Verification items for the finished model (mm, model axes). Give positions to 0.01 mm unless a question says otherwise; leave off trailing zeros. Order: outer loops, then holes, each group sorted by start corner. A loop starts at its lowest first (then second) coordinate and runs counter-clockwise, first axis right, second up. Notation, with made-up numbers: M 10,86 L 38,86 A29 ccw 38,109 Z; hole C 59.25,43 d9. An arc over 180 degrees is marked long. Answer as a JSON object with one key per item and string values.
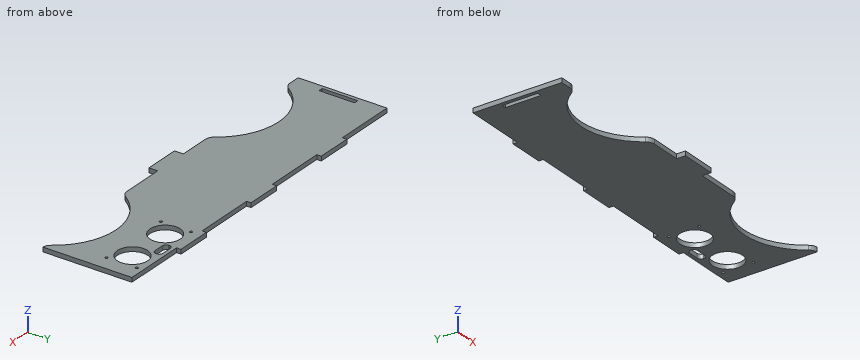
```python
from build123d import *

# Parameters (mm, degrees)
SKETCH1_R           = 8.5
SKETCH1_R_2         = 0.75
SKETCH1_W           = 2.5
SKETCH1_H           = 20
BOSS_EXTRUDE1_DEPTH = 1.25
FILLET2_R           = 5


with BuildPart() as part:
    # Sketch1 → Boss-Extrude1 (new, symmetric)
    with BuildSketch(Plane.XY):
        with BuildLine():
            Line((-100, -25), (-100, 25))
            Line((-100, 25), (-65, 25))
            Line((-65, 25), (-65, 27.5))
            Line((-65, 27.5), (-45, 27.5))
            Line((-45, 27.5), (-45, 25))
            Line((-45, 25), (-10, 25))
            Line((-10, 25), (-10, 27.5))
            Line((-10, 27.5), (10, 27.5))
            Line((10, 27.5), (10, 25))
            Line((10, 25), (45, 25))
            Line((45, 25), (45, 27.5))
            Line((45, 27.5), (65, 27.5))
            Line((65, 27.5), (65, 25))
            Line((65, 25), (100, 25))
            Line((100, 25), (100, -25))
            Line((100, -25), (97.62, -25))
            ThreePointArc((97.62, -25), (67.309110868, -7.5), (36.998221735, -25))
            Line((36.998221735, -25), (10, -25))
            Line((10, -25), (10, -30))
            Line((10, -30), (-10, -30))
            Line((-10, -30), (-10, -25))
            Line((-10, -25), (-30.118221735, -25))
            ThreePointArc((-30.118221735, -25), (-60.429110868, -7.5), (-90.74, -25))
            Line((-90.74, -25), (-100, -25))
        make_face()
        with Locations((57.2, 13)):
            Circle(SKETCH1_R, mode=Mode.SUBTRACT)
        with Locations((48.75, 4.5)):
            Circle(SKETCH1_R_2, mode=Mode.SUBTRACT)
        with Locations(Location((91.25, 4.5, 0), (0, 0, 180))):
            Circle(SKETCH1_R_2, mode=Mode.SUBTRACT)
        with Locations(Location((82.8, 13, 0), (0, 0, 180))):
            Circle(SKETCH1_R, mode=Mode.SUBTRACT)
        with Locations((91.25, 21.5)):
            Circle(SKETCH1_R_2, mode=Mode.SUBTRACT)
        with Locations(Location((48.75, 21.5, 0), (0, 0, 180))):
            Circle(SKETCH1_R_2, mode=Mode.SUBTRACT)
        with Locations((-96.75, 0)):
            Rectangle(SKETCH1_W, SKETCH1_H, mode=Mode.SUBTRACT)
        with BuildLine():
            Line((67, 18.6), (73, 18.6))
            ThreePointArc((73, 18.6), (74.414213562, 19.185786438), (75, 20.6))
            Line((75, 20.6), (75, 21))
            ThreePointArc((75, 21), (74.414213562, 22.414213562), (73, 23))
            Line((73, 23), (67, 23))
            ThreePointArc((67, 23), (65.585786438, 22.414213562), (65, 21))
            Line((65, 21), (65, 20.6))
            ThreePointArc((65, 20.6), (65.585786438, 19.185786438), (67, 18.6))
        make_face(mode=Mode.SUBTRACT)
    extrude(amount=BOSS_EXTRUDE1_DEPTH, both=True)

    # Fillet2
    # the kernel refuses this fillet: 5 mm, written as the material it takes off along each edge
    with BuildSketch(Plane(origin=(97.62, -25, 7.66613531), x_dir=(-0.5314154668172085, 0.8471113277648036, 0), z_dir=(0, 0, -1))) as fillet2_piece_1:
        with BuildLine():
            CenterArc((2.749772276, 4.996638315), FILLET2_R, 216.591278999, 51.307578807)
            Line((-1.264768811, 2.01612496), (-1.345059633, 1.956514693))
            ThreePointArc((-1.345059633, 1.956514693), (-0.717095538, 0.954920933), (-0.084711133, -0.053141547))
            Line((-0.084711133, -0.053141547), (0.003666363, -0.099932766))
            ThreePointArc((0.003666363, -0.099932766), (1.283227062, -0.076468208), (2.562787761, -0.099932766))
            Line((2.562787761, -0.099932766), (2.566454124, 0))
        make_face()
    extrude(amount=15.332270621, mode=Mode.SUBTRACT)
    with BuildSketch(Plane(origin=(36.998221735, -25, 8.15250564), x_dir=(-1, 0, 0), z_dir=(0, 0, -1)), Plane(origin=(-30.118221735, -25, -8.15250564), x_dir=(1, 0, 0), z_dir=(0, 0, 1))) as fillet2_piece_2:
        with BuildLine():
            CenterArc((2.761002256, 5), FILLET2_R, 214.228866328, 55.771133672)
            Line((-1.372984168, 2.1875), (-1.455663896, 2.13125))
            ThreePointArc((-1.455663896, 2.13125), (-0.751006819, 1.053257332), (-0.08660254, -0.05))
            Line((-0.08660254, -0.05), (0, -0.1))
            Line((0, -0.1), (2.761002256, -0.1))
            Line((2.761002256, -0.1), (2.761002256, 0))
        make_face()
    extrude(amount=16.305011279, mode=Mode.SUBTRACT)
    with BuildSketch(Plane(origin=(-90.74, -25, -8.15250564), x_dir=(-1, 0, 0), z_dir=(0, 0, 1))) as fillet2_piece_3:
        with BuildLine():
            CenterArc((2.761002256, -5), FILLET2_R, 90, 55.771133672)
            Line((-1.372984168, -2.1875), (-1.455663896, -2.13125))
            ThreePointArc((-1.455663896, -2.13125), (-0.751006819, -1.053257332), (-0.08660254, 0.05))
            Line((-0.08660254, 0.05), (0, 0.1))
            Line((0, 0.1), (2.761002256, 0.1))
            Line((2.761002256, 0.1), (2.761002256, 0))
        make_face()
    extrude(amount=16.305011279, mode=Mode.SUBTRACT)


solid = part.part
```
Q1. Material ranges on L1, parallel to X at y = -15, z = -0.7; L2, parallel to X at y = -22.5, z = -0.4; L3, parallel to Y at x = 13, z = -0.1, recorded low to high.
Resolved:
{"L1": "x = -100 to -82.08, -38.78 to 45.66, 88.96 to 100", "L2": "x = -100 to -89.15, -31.71 to 38.59, 96.03 to 100", "L3": "y = -25 to 25"}
Q2. Section check B-B on x = 82.8. Record the cut outline in (y, z).
Resolved:
{"outline": "M -11.11,-1.25 L 4.5,-1.25 L 4.5,1.25 L -11.11,1.25 Z; M 21.5,-1.25 L 25,-1.25 L 25,1.25 L 21.5,1.25 Z"}
Q3. Section check C-C on z = -0.3. Count the separate pieces of the cut face and the enclosed holes in it, then the cut area to 3 significant figures.
Resolved:
{"separate pieces": "1", "enclosed holes": "8", "area": "8,190 mm²"}
Q4. Section check A-A on y = 13. Record the cut outline in (x, z), then the cut area to 3 significant figures.
Resolved:
{"outline": "M -100,-1.25 L 48.7,-1.25 L 48.7,1.25 L -100,1.25 Z; M 65.7,-1.25 L 74.3,-1.25 L 74.3,1.25 L 65.7,1.25 Z; M 91.3,-1.25 L 100,-1.25 L 100,1.25 L 91.3,1.25 Z", "area": "415 mm²"}
Q5. Section check D-D on y = -20. Record the cut outline in (x, z).
Resolved:
{"outline": "M -100,-1.25 L -87.24,-1.25 L -87.24,1.25 L -100,1.25 Z; M -33.62,-1.25 L 40.5,-1.25 L 40.5,1.25 L -33.62,1.25 Z; M 94.12,-1.25 L 100,-1.25 L 100,1.25 L 94.12,1.25 Z"}
Q6. Gauge pin test, flat end, axial feed: pin 1 Ø0.8 at (x, z) = (-32.5, 0.5) entering from +Y. Record the tip position at first contact, or that the pin passes through.
Resolved:
{"pin 1": "stops at y = 25"}
